from build123d import *

# Parameters (mm, degrees)
SKETCH1_W           = 150
SKETCH1_H           = 30
BOSS_EXTRUDE1_DEPTH = 5
CUT_EXTRUDE1_DEPTH  = 78.136243103


with BuildPart() as part:
    # Sketch1 → Boss-Extrude1 (new, symmetric)
    with BuildSketch(Plane(origin=(0, 0, 0), x_dir=(1, 0, 0), z_dir=(0, 1, 0))):
        Rectangle(SKETCH1_W, SKETCH1_H)
    extrude(amount=BOSS_EXTRUDE1_DEPTH, both=True)

    # Sketch2 → Cut-Extrude1 (cut, through all)
    with BuildSketch(Plane(origin=(0, 5, 0), x_dir=(1, 0, 0), z_dir=(0, 1, 0))):
        with BuildLine():
            Line((-65.35, 6.708203932), (-65.35, -6.708203932))
            ThreePointArc((-65.35, -6.708203932), (-57.6, -10.25), (-49.85, -6.708203932))
            Line((-49.85, -6.708203932), (-49.85, 6.708203932))
            ThreePointArc((-49.85, 6.708203932), (-57.6, 10.25), (-65.35, 6.708203932))
        make_face()
    cut_extrude1 = extrude(amount=-CUT_EXTRUDE1_DEPTH, mode=Mode.SUBTRACT)

    # Mirror1: Cut-Extrude1 across plane
    add(cut_extrude1.mirror(Plane(origin=(0, 0, 0), x_dir=(0, 0, 1), z_dir=(1, 0, 0))), mode=Mode.SUBTRACT)


solid = part.part
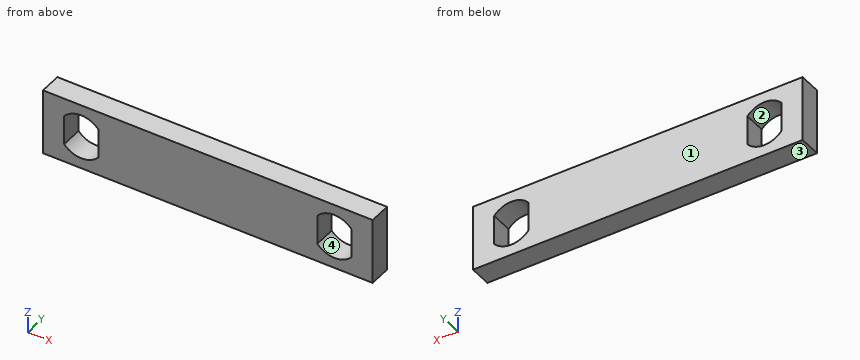
Source: CAD feature listing. Evaluate the final solid. Frame: model axes, mm. Face numbers are marked on the shaded views. A direction names the side the tool comes from. Give positions to 0.01 mm unless a question says otherwise; leave off trailing zeros. Write each loop counter-clockwise with the first axis right and the second up, starting at its lowest first coordinate (ties: lowest second). Pieces come first, ordered by that corner, then holes. Notation, with made-up numbers: M -3,-30.5 L 37,-30.5 A23 cw 37,-7.5 Z; hole C 15.5,68.25 d3. An arc over 180 degrees is marked long. Return JSON: item names as keys, results as strings. Group by question number.
1) Cut plane B-B, the plane y = 1.75. Output: boundary loops of the cut face in (x, z), then the cut area to 3 significant figures.
2) Set-up query: the marked faces 3 and 4. Return all of +Z, -Z, +X, -X, +Y, -Y with unobstructed straight access to the full face (end or side cutting, diameter ignored); none if empty.
3) Cut plane D-D, the plane z = 9. Output: boundary loops of the cut face in (x, y), then the cut area to 3 significant figures.
4) Cut plane C-C, the plane x = 58. Output: boundary loops of the cut face in (y, z).
5) Draft query along X for the marked faces 1 and 2. Return one class per face: released by +X, released by -X, zero draft, split by the parting line, or undercut.
6) Cut plane A-A, the plane z = -2.75. Output: boundary loops of the cut face in (x, y).
7) Ray query, L1, parallel to X at y = 1.5, z = -5; L2, parallel to X at y = 2, z = 9; L3, parallel to Z at x = -56, y = -1.5. Return the intervals inside material, ascending.
Data:
{
 "1": {"outline": "M -75,-15 L 75,-15 L 75,15 L -75,15 Z; hole M -65.35,-6.71 A10.25 ccw -49.85,-6.71 L -49.85,6.71 A10.25 ccw -65.35,6.71 Z; hole M 49.85,-6.71 A10.25 ccw 65.35,-6.71 L 65.35,6.71 A10.25 ccw 49.85,6.71 Z", "area": "3,930 mm²"},
 "2": {"face 3": "-Z, +X, -X, +Y, -Y", "face 4": "+Y, -Y"},
 "3": {"outline": "M -75,-5 L -62.51,-5 L -62.51,5 L -75,5 Z; M -52.69,-5 L 52.69,-5 L 52.69,5 L -52.69,5 Z; M 62.51,-5 L 75,-5 L 75,5 L 62.51,5 Z", "area": "1,300 mm²"},
 "4": {"outline": "M -5,-15 L 5,-15 L 5,-10.24 L -5,-10.24 Z; M -5,10.24 L 5,10.24 L 5,15 L -5,15 Z"},
 "5": {"face 1": "zero draft", "face 2": "undercut"},
 "6": {"outline": "M -75,-5 L -65.35,-5 L -65.35,5 L -75,5 Z; M -49.85,-5 L 49.85,-5 L 49.85,5 L -49.85,5 Z; M 65.35,-5 L 75,-5 L 75,5 L 65.35,5 Z"},
 "7": {"L1": "x = -75 to -65.35, -49.85 to 49.85, 65.35 to 75", "L2": "x = -75 to -62.51, -52.69 to 52.69, 62.51 to 75", "L3": "z = -15 to -10.12, 10.12 to 15"}
}
